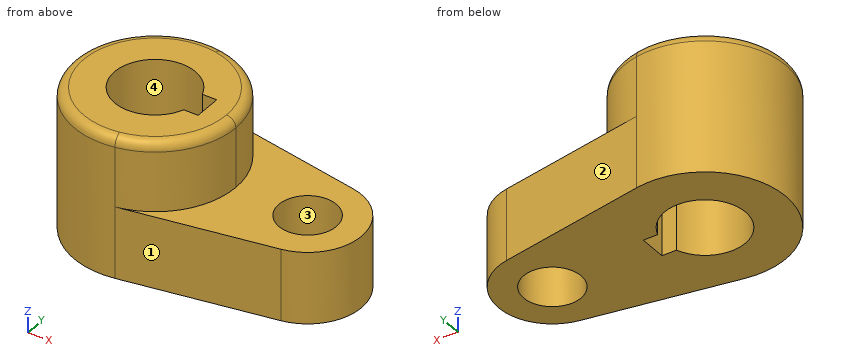
from build123d import *

# Parameters (mm, degrees)
F0_R     = 10.16
F1_DEPTH = 25.4
F3_DEPTH = 24.4602
F4_R     = 3.302


with BuildPart() as f1:
    # F0 (on Top) → F1 (new body)
    with BuildSketch(Plane.XY):
        with BuildLine():
            ThreePointArc((5.042647, 28.126541), (21.916025, 18.336262), (28.575, 0))
            ThreePointArc((28.575, 0), (21.916025, -18.336261), (5.042648, -28.126541))
            Line((5.042648, -28.126541), (57.336765, -18.751028))
            ThreePointArc((57.336765, -18.751028), (73.025, 0), (57.336765, 18.751028))
            Line((57.336765, 18.751028), (5.042647, 28.126541))
        make_face()
        with Locations((53.975, 0)):
            Circle(F0_R, mode=Mode.SUBTRACT)
        with BuildLine():
            ThreePointArc((5.042648, -28.126541), (21.916025, -18.336261), (28.575, 0))
            ThreePointArc((28.575, 0), (21.916025, 18.336262), (5.042647, 28.126541))
            ThreePointArc((5.042647, 28.126541), (-28.575, 0), (5.042648, -28.126541))
        make_face()
        with BuildLine():
            ThreePointArc((13.447765, -4.826), (-14.2875, 0), (13.447765, 4.826))
            Line((13.447765, 4.826), (18.5293, 4.826))
            Line((18.5293, 4.826), (18.5293, 0))
            Line((18.5293, 0), (18.5293, -4.826))
            Line((18.5293, -4.826), (13.447765, -4.826))
        make_face(mode=Mode.SUBTRACT)
    extrude(amount=F1_DEPTH)

    # F2 (on face) → F3 (join)
    with BuildSketch(Plane.XY.offset(25.4)):
        with BuildLine():
            ThreePointArc((5.042648, -28.126541), (21.916025, -18.336261), (28.575, 0))
            ThreePointArc((28.575, 0), (21.916025, 18.336262), (5.042647, 28.126541))
            ThreePointArc((5.042647, 28.126541), (-28.575, 0), (5.042648, -28.126541))
        make_face()
        with BuildLine():
            ThreePointArc((13.447765, -4.826), (-14.2875, 0), (13.447765, 4.826))
            Line((13.447765, 4.826), (18.5293, 4.826))
            Line((18.5293, 4.826), (18.5293, -4.826))
            Line((18.5293, -4.826), (13.447765, -4.826))
        make_face(mode=Mode.SUBTRACT)
    extrude(amount=F3_DEPTH)

    # F4
    f4_edges = [f1.edges().sort_by_distance(p)[0] for p in [
        (-5.042648, 28.126541, 49.8602),
    ]]
    fillet(f4_edges, radius=F4_R)


solid = f1.part
Build history of the part. All positions in model axes, mm. Face numbers are marked on the shaded views. Give positions to 0.01 mm unless a question says otherwise; leave off trailing zeros. Loops run counter-clockwise (first coordinate to the right, second up) from the corner with the lowest first, then second, coordinate; pieces in that order, holes last. Notation, with made-up numbers: (-22.75, 71.5) - (20.25, 71.5) arc R6 ccw to (20.25, 81.5) - close; hole circle Ø6 at (58.5, -19.5). An arc over 180 degrees is marked (long way). Write item = value, one per line. Start each with the question number.
1) Probe probe 1 along Y at (x, z) = (0, 24.5) (1 decimal); probe 2 along X at (y, z) = (3, 21); probe 3 along X at (y, z) = (0, 33) (1 decimal). List the from-to ranges inside material, lowest first. Write a range as from..to.
2) Band-saw the part on B-B on y = 9. Count the separate pieces of the cut face and the enclosed holes in it, plus the area to 3 significant figures.
3) Drop flat-ended pins along their axis: pin 1 Ø5 at (x, z) = (18, 29.5) entering from +Y; pin 2 Ø6 at (y, z) = (5, 9) entering from -X; pin 3 Ø3 at (y, z) = (-2, 17) entering from -X; pin 4 Ø12 at (x, y) = (-17.5, 22) entering from -Z. Give the stop position or say it passes through.
4) Pull direction Y, two halves, no side cores. Call the marked faces 1, 2, 3 and 4: +Y half, -Y half, draft (parallel to the pull), parting line (faces both ways), or undercut.
5) Band-saw the part on C-C on x = 36.5. Give the cut face in (y, z), plus the area to 3 significant figures.
Final values:
q1.probe_1 = -28.6..-14.3, 14.3..28.6
q1.probe_2 = -28.42..-13.97, 18.53..44.27, 63.68..72.79
q1.probe_3 = -28.6..-14.3, 18.5..28.6
q2.separate_pieces = 3
q2.enclosed_holes = 0
q2.area = 2,460 mm²
q3.pin_1 = 24.01
q3.pin_2 = -28.5
q3.pin_3 = -28.57
q3.pin_4 = 0
q4.face_1 = -Y half
q4.face_2 = +Y half
q4.face_3 = undercut
q4.face_4 = undercut
q5.outline = (-22.49, 0) - (22.49, 0) - (22.49, 25.4) - (-22.49, 25.4) - close
q5.area = 1,140 mm²
